Autodesk Inventor part; units mm, degrees
ref_plane "YZ Plane" through (0, 0, 0) normal (1, 0, 0) x (0, 1, 0)
ref_plane "XZ Plane" through (0, 0, 0) normal (0, 1, 0) x (-1, 0, 0)
ref_plane "XY Plane" through (0, 0, 0) normal (0, 0, 1) x (1, 0, 0)
sketch "Sketch2" plane through (0, 0, 0) normal (0, 0, 1) x (1, 0, 0)
  line L0 (0, 0) -> (12.7, 0)
  line L1 (0, 0) -> (0, 12.7)
  arc A0 (12.7, 0) -> (0, 12.7) centre (0, 0) ccw
  circle A1 centre (5.08, 5.08) radius 3.1115
  dimension "d4" = 12.7
  dimension "d5" = 6.223
  dimension "d6" = 5.08
  dimension "d7" = 5.08
extrude "Extrusion1" add sketch "Sketch2" along normal blind 3.81
sketch "Sketch4" plane through (0, 0, 0) normal (0, 0, -1) x (-1, 0, 0)
  arc A0 (0, 12.7) -> (-12.7, 0) centre (0, 0) ccw
  line L0 (-12.7, 0) -> (-12.7, -1.27)
  line L1 (0, 12.7) -> (1.27, 12.7)
  line L2 (2.54, 11.43) -> (2.54, -1.27)
  line L3 (1.27, -2.54) -> (-11.43, -2.54)
  line L4 (0, 12.7) -> (0, 0)
  line L5 (0, 0) -> (-12.7, 0)
  arc A1 (-12.7, -1.27) -> (-11.43, -2.54) centre (-11.43, -1.27) ccw
  arc A2 (1.27, -2.54) -> (2.54, -1.27) centre (1.27, -1.27) ccw
  arc A3 (2.54, 11.43) -> (1.27, 12.7) centre (1.27, 11.43) ccw
  point P0 (-12.7, -2.54)
  point P1 (2.54, 12.7)
  dimension "d10" = 2.54
  dimension "d11" = 2.54
  dimension "d12" = 1.27
extrude "Extrusion2" add sketch "Sketch4" along normal blind 3.048 and the other way blind 3.81 contours L1 A3 L2 A2 L3 A1 L0 L5 L4
sketch "Sketch5" plane through (0, 0, 3.81) normal (0, 0, 1) x (1, 0, 0)
  line L0 (-1.27, -2.54) -> (11.43, -2.54)
  line L1 (-2.54, -1.27) -> (-2.54, 11.43)
  arc A0 (12.7, 0) -> (0, 12.7) centre (0, 0) ccw
  line L2 (0, 12.7) -> (-1.27, 12.7)
  line L3 (12.7, 0) -> (12.7, -1.27)
  arc A1 (-1.27, 12.7) -> (-2.54, 11.43) centre (-1.27, 11.43) ccw
  arc A2 (-2.54, -1.27) -> (-1.27, -2.54) centre (-1.27, -1.27) ccw
  arc A3 (11.43, -2.54) -> (12.7, -1.27) centre (11.43, -1.27) ccw
  line L4 (0, 12.7) -> (0, 0)
  line L5 (0, 0) -> (12.7, 0)
  circle A4 centre (5.08, 5.08) radius 3.1115
  dimension "d17" = 1.27
  dimension "d18" = 2.54
  dimension "d19" = 2.54
extrude "Extrusion3" add sketch "Sketch5" along normal blind 2.794 contours A2 L1 A1 L2 L4 L5 L3 A3 L0 | L5 L4 A0 | A4
sketch "Sketch7" plane through (-1.27, -2.54, -3.048) normal (0, -1, 0) x (1, 0, 0)
  line L0 (12.7, 0) -> (12.7, 9.652)
  line L1 (12.7, 9.652) -> (6.3503, 17.5834)
  line L2 (0, 9.652) -> (0, 0)
  line L3 (0, 9.652) -> (-1.3892, 11.3873)
  line L4 (6.3503, 17.5834) -> (-1.3892, 11.3873)
  line L5 (12.7, 9.652) -> (0, 9.652)
  point P0 (1.27, 3.048)
  dimension "d22" = 141.32
  dimension "d23" = 141.32
  dimension "d24" = 10.16
extrude "Extrusion4" add sketch "Sketch7" against normal blind 12.7
sketch "Sketch8" plane through (5.0803, -2.54, 14.5354) normal (-0.6249702, 0, 0.7806486) x (0.7806486, 0, 0.6249702)
  line L0 (0, 0) -> (-9.9142, 0) construction
  line L1 (-9.9142, 12.7) -> (0, 12.7) construction
  line L2 (0, 0) -> (-9.9142, 12.7) construction
  line L3 (-9.9142, 0) -> (-9.9142, 12.7) construction
  line L4 (-9.9142, 0) -> (-1.8469, 10.3341) construction
  circle A0 centre (-4.9571, 6.35) radius 2
  point P0 (-13.0501, 2.54)
  dimension "d27" = 4
extrude "Extrusion5" cut sketch "Sketch8" against normal blind 7
fillet "Fillet1" radius 7.62 1 edges at (8.2552, 10.16, 10.5697)
equation "\"d27\" = m3_heat_set_insert"
equation "\"d28\" = m3_heat_set_depth"
equation "\"m3_heat_set_insert\" = 4"
equation "\"m3_clearance\" = 3.4"
equation "\"m3_heat_set_depth\" = 7"
equation "\"robot_diameter\" = 354"
equation "\"hardboard_thickness\" = 5"
properties part number "display_bottom_support_left"
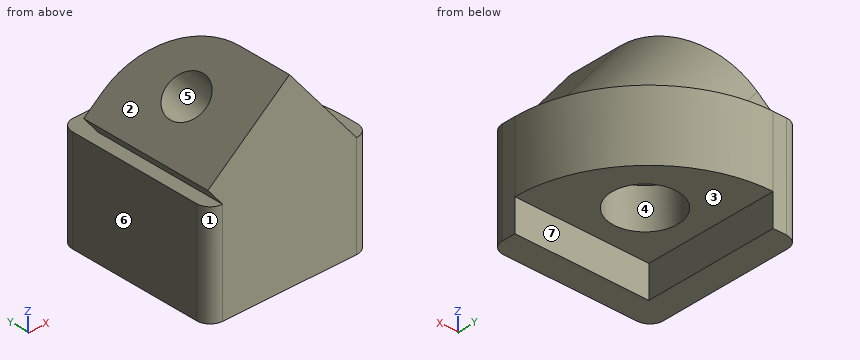
Build history of the part. All positions in model axes, mm. Face numbers are marked on the shaded views. A direction names the side the tool comes from. Give positions to 0.01 mm unless a question says otherwise; leave off trailing zeros. Loops run counter-clockwise (first coordinate to the right, second up) from the corner with the lowest first, then second, coordinate; pieces in that order, holes last.
Item 1: Pull direction Y, two halves, no side cores. Call the marked faces 4, 5, 6 and 7: released by +Y, released by -Y, zero draft, split by the parting line, or undercut.
Answers follow:
face 4: undercut
face 5: undercut
face 6: zero draft
face 7: released by +Y
Item 2: Slice it at A-A, the plane y = 5.08. List the corners of the cut face in (x, z).
Answers follow:
outline: (-2.66, 8.34) - (-1.27, 6.6) - (-2.54, 6.6) - (-2.54, -3.05) - (0, -3.05) - (0, 0) - (1.97, 0) - (1.97, 3.81) - (8.19, 3.81) - (8.19, 0) - (11.64, 0) - (11.64, 6.6) - (10.87, 6.6) - (4.74, 14.26) - (2.42, 12.4) - (6.79, 6.94) - (4.38, 5.01) - (0, 10.47) - close
Item 3: Flat gauge pins, fed straight in: pin 1 (1.5 mm diameter, centred on x = -1, y = 0.5, fed in from +Z); pin 2 (1 mm diameter, centred on x = 5.5, y = 1.5, fed in from -Z); pin 3 (2.5 mm diameter, centred on x = 6, z = -1, fed in from +Y). Where does each tip first touch, or does it go through?
Answers follow:
pin 1: stops at z = 10.27
pin 2: stops at z = 0
pin 3: stops at y = 11.56
Item 4: Slice it at B-B, the plane y = 6.75. List the corners of the cut face in (x, z), and give its area (3 significant figures).
Answers follow:
outline: (-2.66, 8.34) - (-1.27, 6.6) - (-2.54, 6.6) - (-2.54, -3.05) - (0, -3.05) - (0, 0) - (2.45, 0) - (2.45, 3.81) - (7.71, 3.81) - (7.71, 0) - (10.76, 0) - (10.76, 6.6) - (9.8, 6.6) - (4.09, 13.74) - close
area: 125 mm2
Item 5: Which spindle directions (+Z, -Z, +X, -X, +Y, -Y) get a long thin tool onto all of the face, cutting with end or side? Do the marked faces 1, 2 and 3. Say none if no direction does.
Answers follow:
face 1: -Z, -X, -Y
face 2: +Z, -X, +Y, -Y
face 3: -Z, +X, +Y
Item 6: Drill centre lines: line 1 (Z direction, x = 3, y = 3.25); line 2 (Y direction, x = 7.5, z = 3.75); line 3 (Z direction, x = 1.75, y = 10.25). Where is each one in solid material? Low to high.
Answers follow:
line 1: z = 3.81 to 6.13, 12.27 to 12.87
line 2: y = -2.54 to 3.12, 7.04 to 10.25
line 3: z = 0 to 6.6
